Can you work these out from the model? Positions are in its coordinate system, mm. Coordinates: 2 decimals unless noted, no trailing zeros. Order: outer loops, then holes, each group sorted by start corner. A loop starts at its lowest first (then second) coordinate and runs counter-clockwise, first axis right, second up. Notation, with made-up numbers: (-23.75, -40) -> (33.25, -40) arc R20 ccw to (33.25, -4) -> close; hole circle Ø1 at (25.25, 80). An arc over 180 degrees is marked (long way). Answer in a Markdown table with one row per item.
```python
from build123d import *

# Parameters (mm, degrees)
SKETCH1_R           = 2.4
BOSS_EXTRUDE1_DEPTH = 150


with BuildPart() as part:
    # Sketch1 → Boss-Extrude1 (new body)
    with BuildSketch(Plane(origin=(0, 0, 0), x_dir=(1, 0, 0), z_dir=(0, 1, 0))):
        with BuildLine():
            ThreePointArc((-10, -9), (-9.707106781, -9.707106781), (-9, -10))
            Line((-9, -10), (-3.1, -10))
            Line((-3.1, -10), (-3.1, -8.7))
            ThreePointArc((-3.1, -8.7), (-3.246446609, -8.346446609), (-3.6, -8.2))
            Line((-3.6, -8.2), (-5.5, -8.2))
            Line((-5.5, -8.2), (-5.5, -6.376528763))
            Line((-5.5, -6.376528763), (-3.123471237, -4))
            Line((-3.123471237, -4), (0, -4))
            Line((0, -4), (3.123471237, -4))
            Line((3.123471237, -4), (5.5, -6.376528763))
            Line((5.5, -6.376528763), (5.5, -8.2))
            Line((5.5, -8.2), (3.6, -8.2))
            ThreePointArc((3.6, -8.2), (3.246446609, -8.346446609), (3.1, -8.7))
            Line((3.1, -8.7), (3.1, -10))
            Line((3.1, -10), (9, -10))
            ThreePointArc((9, -10), (9.707106781, -9.707106781), (10, -9))
            Line((10, -9), (10, -3.1))
            Line((10, -3.1), (8.7, -3.1))
            ThreePointArc((8.7, -3.1), (8.346446609, -3.246446609), (8.2, -3.6))
            Line((8.2, -3.6), (8.2, -5.5))
            Line((8.2, -5.5), (6.376528763, -5.5))
            Line((6.376528763, -5.5), (4, -3.123471237))
            Line((4, -3.123471237), (4, 0))
            Line((4, 0), (4, 3.123471237))
            Line((4, 3.123471237), (6.376528763, 5.5))
            Line((6.376528763, 5.5), (8.2, 5.5))
            Line((8.2, 5.5), (8.2, 3.6))
            ThreePointArc((8.2, 3.6), (8.346446609, 3.246446609), (8.7, 3.1))
            Line((8.7, 3.1), (10, 3.1))
            Line((10, 3.1), (10, 9))
            ThreePointArc((10, 9), (9.707106781, 9.707106781), (9, 10))
            Line((9, 10), (3.1, 10))
            Line((3.1, 10), (3.1, 8.7))
            ThreePointArc((3.1, 8.7), (3.246446609, 8.346446609), (3.6, 8.2))
            Line((3.6, 8.2), (5.5, 8.2))
            Line((5.5, 8.2), (5.5, 6.376528763))
            Line((5.5, 6.376528763), (3.123471237, 4))
            Line((3.123471237, 4), (0, 4))
            Line((0, 4), (-3.123471237, 4))
            Line((-3.123471237, 4), (-5.5, 6.376528763))
            Line((-5.5, 6.376528763), (-5.5, 8.2))
            Line((-5.5, 8.2), (-3.6, 8.2))
            ThreePointArc((-3.6, 8.2), (-3.246446609, 8.346446609), (-3.1, 8.7))
            Line((-3.1, 8.7), (-3.1, 10))
            Line((-3.1, 10), (-9, 10))
            ThreePointArc((-9, 10), (-9.707106781, 9.707106781), (-10, 9))
            Line((-10, 9), (-10, 3.1))
            Line((-10, 3.1), (-8.7, 3.1))
            ThreePointArc((-8.7, 3.1), (-8.346446609, 3.246446609), (-8.2, 3.6))
            Line((-8.2, 3.6), (-8.2, 5.5))
            Line((-8.2, 5.5), (-6.376528763, 5.5))
            Line((-6.376528763, 5.5), (-4, 3.123471237))
            Line((-4, 3.123471237), (-4, 0))
            Line((-4, 0), (-4, -3.123471237))
            Line((-4, -3.123471237), (-6.376528763, -5.5))
            Line((-6.376528763, -5.5), (-8.2, -5.5))
            Line((-8.2, -5.5), (-8.2, -3.6))
            ThreePointArc((-8.2, -3.6), (-8.346446609, -3.246446609), (-8.7, -3.1))
            Line((-8.7, -3.1), (-10, -3.1))
            Line((-10, -3.1), (-10, -9))
        make_face()
        Circle(SKETCH1_R, mode=Mode.SUBTRACT)
    extrude(amount=BOSS_EXTRUDE1_DEPTH)


solid = part.part
```
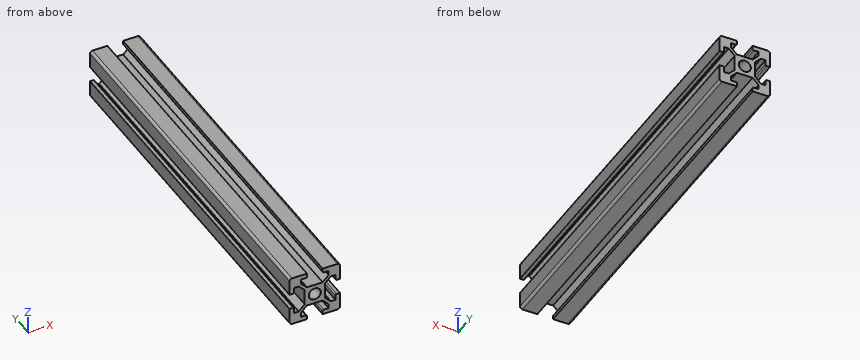
(1) I need wall thicknesses on line 1 (X direction, y = 105.5, z = 8); line 2 (X direction, y = 54, z = 0); line 3 (X direction, y = 46, z = -4.75). Which ranges of each line are inside material? Lowest first, please. Write a range as [from, to].
Response values:
| item | result |
|---|---|
| line 1 | [-10, -5.5], [5.5, 10] |
| line 2 | [-4, -2.4], [2.4, 4] |
| line 3 | [-10, -8.2], [-5.63, -3.87], [3.87, 5.63], [8.2, 10] |
(2) Suppose I cut it at B-B (z = 0). Please give me the cut outline in (x, y).
Response values:
| item | result |
|---|---|
| outline | (-4, 0) -> (-2.4, 0) -> (-2.4, 150) -> (-4, 150) -> close; (2.4, 0) -> (4, 0) -> (4, 150) -> (2.4, 150) -> close |
(3) Will this pin go through, and if not, where does the flat tip stop? pin 1 Ø0.7 at (y, z) = (38.5, -9.5) entering from -X.
Response values:
| item | result |
|---|---|
| pin 1 | x = -9.99 |
(4) Suppose I cut it at A-A (x = 0). Please give me the cut outline in (y, z).
Response values:
| item | result |
|---|---|
| outline | (0, -4) -> (150, -4) -> (150, -2.4) -> (0, -2.4) -> close; (0, 2.4) -> (150, 2.4) -> (150, 4) -> (0, 4) -> close |
